Job drawing, mm, ordinate dimensions from the low corner. One solid piece. Round coordinates to 2 decimals unless told otherwise and drop trailing zeros. Write each loop counter-clockwise with the first axis right and the second up, starting at its lowest first coordinate (ties: lowest second). Pieces come first, ordered by that corner, then holes. Notation, with made-up numbers: (-38, 37.5) -> (4, 37.5) arc R17 cw to (4, 68.5) -> close; hole circle Ø10 at (-3, 59.25). An arc over 180 degrees is marked (long way). Use CSV: the item, a comma, the result in double quotes. Start each with the question number.
(1) Saw through at C-C (y = 7.25). Give the cut face in (x, z), plus the area to 3 significant figures.
(2) Saw through at A-A (z = 60). Give the cut face in (x, y).
(3) Drop flat-ended pins along their axis: pin 1 (1 mm diameter, centred on x = 25.5, y = 4.5, fed in from +Z); pin 2 (1.5 mm diameter, centred on x = 38, y = 8, fed in from +Z); pin 3 (0.6 mm diameter, centred on x = 25.5, y = 5, fed in from -Z). Give the stop position or say it passes through.
(4) Probe line 1 (Z direction, x = 25, y = 6.25); line 2 (Z direction, x = 25, y = 5.25); line 3 (X direction, y = 6, z = 25). List the from-to ranges inside material, lowest first. Write a range as [from, to].
(5) Saw through at B-B (x = 36.5). Give the cut face in (y, z).
(6) Two-plate mould, pull along Z, no slides. Class the marked faces 1, 2, 3 and 4: released by +Z, released by -Z, zero draft, split by the parting line, or undercut.
(7) Saw through at D-D (z = 30). Give the cut face in (x, y).
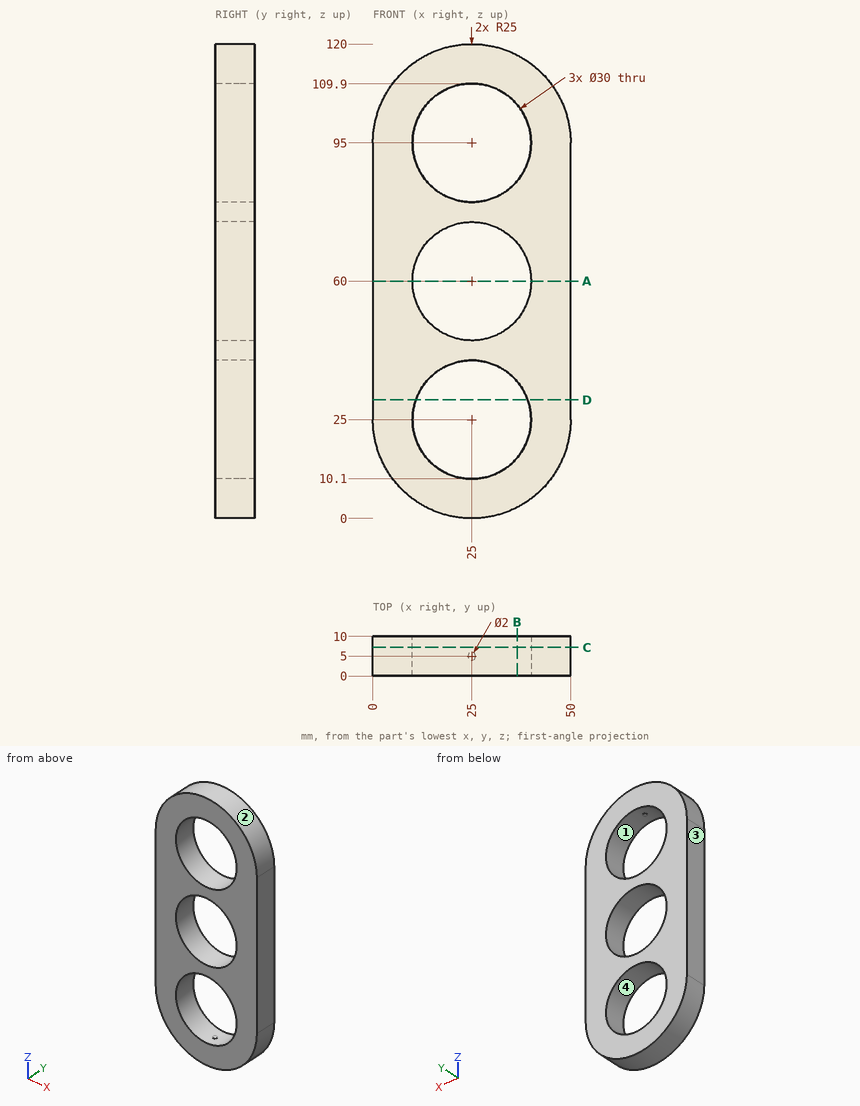
Answers:
1,outline,"(0, 25) arc R25 ccw to (50, 25) -> (50, 95) arc R25 ccw to (0, 95) -> close; hole circle Ø30 at (25, 25); hole circle Ø30 at (25, 60); hole circle Ø30 at (25, 95)"
1,area,"3,340 mm²"
2,outline,"(0, 0) -> (10, 0) -> (10, 10) -> (0, 10) -> close; (40, 0) -> (50, 0) -> (50, 10) -> (40, 10) -> close"
3,pin 1,"stops at z = 120"
3,pin 2,"stops at z = 116.79"
3,pin 3,"stops at z = 0"
4,line 1,"z = [0, 10], [40, 45], [75, 80], [110, 120]"
4,line 2,"z = [0, 10.1], [40, 45], [75, 80], [109.9, 120]"
4,line 3,"x = [0, 10], [40, 50]"
5,outline,"(0, 2.8) -> (10, 2.8) -> (10, 15.37) -> (0, 15.37) -> close; (0, 34.63) -> (10, 34.63) -> (10, 50.37) -> (0, 50.37) -> close; (0, 69.63) -> (10, 69.63) -> (10, 85.37) -> (0, 85.37) -> close; (0, 104.63) -> (10, 104.63) -> (10, 117.2) -> (0, 117.2) -> close"
6,face 1,"undercut"
6,face 2,"released by +Z"
6,face 3,"zero draft"
6,face 4,"undercut"
7,outline,"(0, 0) -> (10.86, 0) -> (10.86, 10) -> (0, 10) -> close; (39.14, 0) -> (50, 0) -> (50, 10) -> (39.14, 10) -> close"
